Input: dimensioned drawing with shaded views. Units: mm. Origin: part minimum x, y, z. Coordinates: 2 decimals unless noted, no trailing zeros. Order: outer loops, then holes, each group sorted by start corner. A loop starts at its lowest first (then second) coordinate and runs counter-clockwise, first axis right, second up.
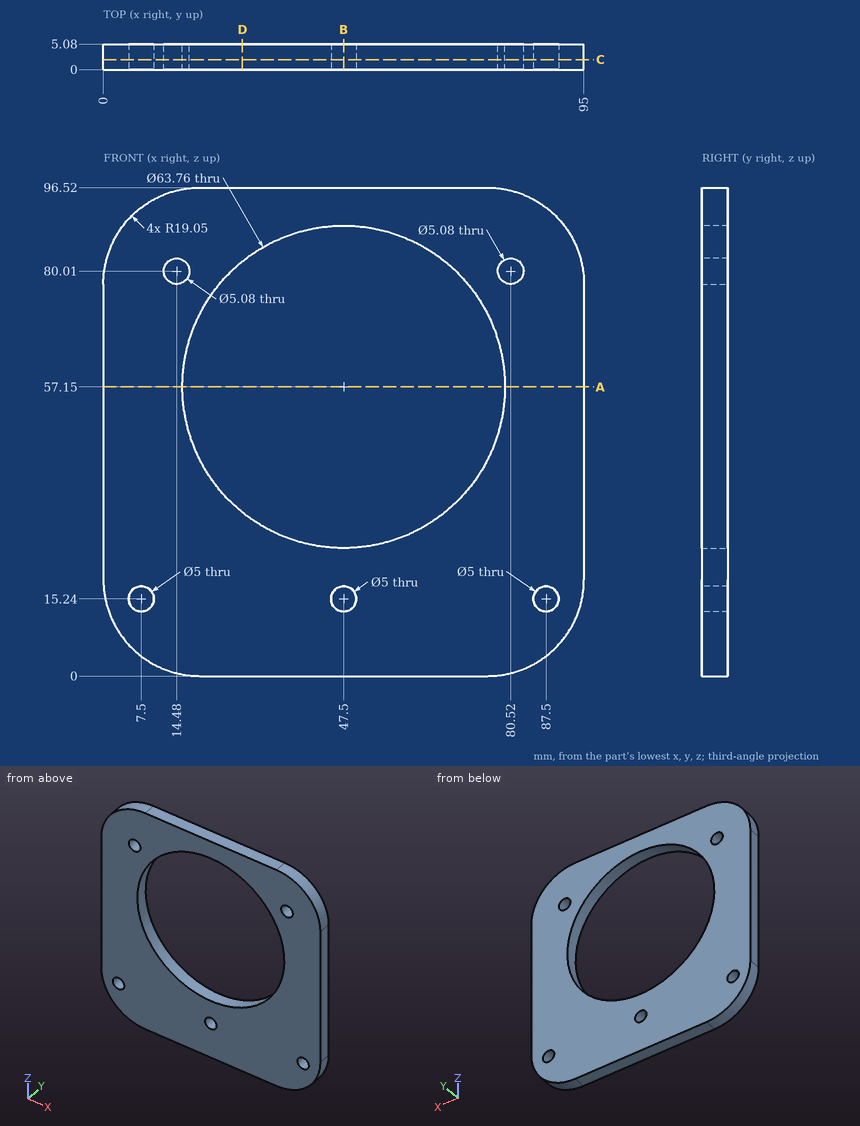
1. Ray query, line 1 (X direction, y = 2.05, z = 81.5); line 2 (X direction, y = 3.95, z = 82); line 3 (Z direction, x = 89, y = 2.75). Return the intervals inside material, ascending.
Findings:
line 1: x = 0.43 to 12.42, 16.54 to 26.92, 68.08 to 78.46, 82.58 to 94.57
line 2: x = 0.55 to 12.9, 16.06 to 27.53, 67.47 to 78.94, 82.1 to 94.45
line 3: z = 5.17 to 13.24, 17.24 to 91.35
2. Section query A-A on z = 57.15. Return loops of the section in (x, y).
Findings:
outline: (0, 0) - (15.62, 0) - (15.62, 5.08) - (0, 5.08) - close; (79.38, 0) - (95, 0) - (95, 5.08) - (79.38, 5.08) - close
3. Section query B-B on x = 47.5. Return loops of the section in (y, z).
Findings:
outline: (0, 0) - (5.08, 0) - (5.08, 12.74) - (0, 12.74) - close; (0, 17.74) - (5.08, 17.74) - (5.08, 25.27) - (0, 25.27) - close; (0, 89.03) - (5.08, 89.03) - (5.08, 96.52) - (0, 96.52) - close
4. Pin query (flat end, axial travel): P1, Ø8, axis at x = 47.5, z = 15.24, coming from the +Y side; P2, Ø1, axis at x = 13, y = 2, coming from the +Z side. Return the tip coordinate at first contact, or that it passes through.
Findings:
P1: stops at y = 5.08
P2: stops at z = 95.69
5. Section query D-D on x = 27.5. Return loops of the section in (y, z).
Findings:
outline: (0, 0) - (5.08, 0) - (5.08, 32.32) - (0, 32.32) - close; (0, 81.98) - (5.08, 81.98) - (5.08, 96.52) - (0, 96.52) - close
6. Section query C-C on y = 2. Return loops of the section in (x, z), plus the area to 3 significant figures.
Findings:
outline: (0, 19.05) arc R19.05 ccw to (19.05, 0) - (75.95, 0) arc R19.05 ccw to (95, 19.05) - (95, 77.47) arc R19.05 ccw to (75.95, 96.52) - (19.05, 96.52) arc R19.05 ccw to (0, 77.47) - close; hole circle Ø5 at (7.5, 15.24); hole circle Ø5.08 at (14.48, 80.01); hole circle Ø63.76 at (47.5, 57.15); hole circle Ø5 at (47.5, 15.24); hole circle Ø5.08 at (80.52, 80.01); hole circle Ø5 at (87.5, 15.24)
area: 5,570 mm2
